```python
from build123d import *

# Parameters (mm, degrees)
ESQUISSE1_R             = 2
BOSS_EXTRU_1_DEPTH      = 5
ESQUISSE2_W             = 12
ESQUISSE2_H             = 2.5
BOSS_EXTRU_2_DEPTH      = 10
BOSS_EXTRU_2_2_DEPTH    = 10
ESQUISSE5_W             = 1.920676926
ESQUISSE5_H             = 10
BOSS_EXTRU_4_DEPTH      = 6.1
ESQUISSE7_W             = 2.5
ESQUISSE7_H             = 10
BOSS_EXTRU_6_DEPTH      = 1.920676926
CONG_4_RADIUS           = 5
CONG_4_LENGTH           = 2.5
BOSS_EXTRU_5_DEPTH      = 10
ESQUISSE4_R             = 2
ENL_V_MAT_EXTRU_2_DEPTH = 27.8404319
CONG_5_RADIUS           = 5
CONG_5_LENGTH           = 2.5


with BuildPart() as part:
    # Esquisse1 → Boss.-Extru.1 (new body)
    with BuildSketch(Plane.XY):
        with BuildLine():
            Line((-15, 5), (10, 5))
            Line((10, 5), (10, -5))
            Line((10, -5), (-15, -5))
            ThreePointArc((-15, -5), (-20, 0), (-15, 5))
        make_face()
        with Locations((-15, 0)):
            Circle(ESQUISSE1_R, mode=Mode.SUBTRACT)
    extrude(amount=BOSS_EXTRU_1_DEPTH)

    # Esquisse5 → Boss.-Extru.4 (add)
    with BuildSketch(Plane.XY.offset(-0.55)):
        with Locations((10.960338463, 0)):
            Rectangle(ESQUISSE5_W, ESQUISSE5_H)
    extrude(amount=BOSS_EXTRU_4_DEPTH)



with BuildPart() as body_2:
    # Esquisse2 → Boss.-Extru.2 (new, through all)
    with BuildSketch(Plane(origin=(0, 5, 0), x_dir=(1, 0, 0), z_dir=(0, 1, 0))):
        with Locations((17.920676926, 1.8)):
            Rectangle(ESQUISSE2_W, ESQUISSE2_H)
    extrude(amount=-BOSS_EXTRU_2_DEPTH)


with BuildPart() as body_3:
    # Esquisse2 → Boss.-Extru.2 2 (new, through all)
    with BuildSketch(Plane(origin=(0, 5, 0), x_dir=(1, 0, 0), z_dir=(0, 1, 0))):
        with Locations((17.920676926, -6.8)):
            Rectangle(ESQUISSE2_W, ESQUISSE2_H)
    extrude(amount=-BOSS_EXTRU_2_2_DEPTH)


with BuildPart() as part_1:
    add(part.part)

    add(body_2.part)  # Boss.-Extru.6 merges body 2

    add(body_3.part)  # Boss.-Extru.6 merges body 3
    # Esquisse7 → Boss.-Extru.6 (add)
    with BuildSketch(Plane.ZY.offset(-11.920676926)):
        with Locations((-1.8, 0)):
            Rectangle(ESQUISSE7_W, ESQUISSE7_H)
        with Locations((6.8, 0)):
            Rectangle(ESQUISSE7_W, ESQUISSE7_H)
    extrude(amount=BOSS_EXTRU_6_DEPTH)

    # Congé4: full round fillet: the end face becomes a half cylinder, R = half its width
    cong_4_face = Plane((23.920676926, 0, 6.8), x_dir=(0, 0, 1), z_dir=(1, 0, 0))  # on the end face: x along it, z out of the body
    cong_4_slab = cong_4_face.offset(-CONG_4_RADIUS / 2) * Box(CONG_4_LENGTH, 2 * CONG_4_RADIUS, CONG_4_RADIUS, mode=Mode.PRIVATE)  # the body's end, R deep
    cong_4_round = Plane((18.920676926, 0, 6.8), x_dir=(1, 0, 0), z_dir=(0, 0, 1)) * Cylinder(CONG_4_RADIUS, CONG_4_LENGTH, mode=Mode.PRIVATE)  # its axis R under the face
    add(cong_4_slab - cong_4_round, mode=Mode.SUBTRACT)

    # Esquisse6 → Boss.-Extru.5 (add, through all)
    with BuildSketch(Plane(origin=(0, 5, 0), x_dir=(1, 0, 0), z_dir=(0, 1, 0))):
        Polygon((10, 0), (10, 3.05), (4.799024164, 0), align=None)
        Polygon((4.799024164, -5), (10, -8.05), (10, -5), align=None)
    extrude(amount=-BOSS_EXTRU_5_DEPTH)

    # Esquisse4 → Enlèv. mat.-Extru.2 (cut, through all)
    with BuildSketch(Plane(origin=(0, 0, -3.05), x_dir=(-1, 0, 0), z_dir=(0, 0, -1))):
        with Locations((-18.856076392, 0)):
            Circle(ESQUISSE4_R)
    extrude(amount=-ENL_V_MAT_EXTRU_2_DEPTH, mode=Mode.SUBTRACT)

    # Congé5: full round fillet: the end face becomes a half cylinder, R = half its width
    cong_5_face = Plane((23.920676926, 0, -1.8), x_dir=(0, 0, -1), z_dir=(1, 0, 0))  # on the end face: x along it, z out of the body
    cong_5_slab = cong_5_face.offset(-CONG_5_RADIUS / 2) * Box(CONG_5_LENGTH, 2 * CONG_5_RADIUS, CONG_5_RADIUS, mode=Mode.PRIVATE)  # the body's end, R deep
    cong_5_round = Plane((18.920676926, 0, -1.8), x_dir=(1, 0, 0), z_dir=(0, 0, -1)) * Cylinder(CONG_5_RADIUS, CONG_5_LENGTH, mode=Mode.PRIVATE)  # its axis R under the face
    add(cong_5_slab - cong_5_round, mode=Mode.SUBTRACT)


solid = part_1.part
```
Geometry: final body of the model. Coordinates: model frame, mm. A direction names the side the tool comes from. Round coordinates to 2 decimals unless told otherwise and drop trailing zeros. Write each loop counter-clockwise with the first axis right and the second up, starting at its lowest first coordinate (ties: lowest second). Pieces come first, ordered by that corner, then holes. Notation, with made-up numbers: (85.25, 46.5) -> (131.25, 46.5) arc R7 ccw to (131.25, 56.5) -> close; hole circle Ø7 at (8.5, 24.25). An arc over 180 degrees is marked (long way). Return JSON: item names as keys, results as strings.
Q1. Set-up query: faces 4 (the flat face through (16.5, 0.1, -0.55)), 5 (the flat face through (-7, 0, 5)), 6 (the flat face through (-7, 0, 0)). Return all of +Z, -Z, +X, -X, +Y, -Y with unobstructed straight access to the full face (end or side cutting, diameter ignored); none if empty.
From the geometry:
{"face 4": "+X, +Y, -Y", "face 5": "+Z, -X, +Y, -Y", "face 6": "-Z, -X, +Y, -Y"}
Q2. Section D-D on y = 4. Return the cut outline in (x, z), and give its area (3 significant figures).
From the geometry:
{"outline": "(-18, 0) -> (4.8, 0) -> (10, -3.05) -> (21.92, -3.05) -> (21.92, -0.55) -> (11.92, -0.55) -> (11.92, 5.55) -> (21.92, 5.55) -> (21.92, 8.05) -> (10, 8.05) -> (4.8, 5) -> (-18, 5) -> close", "area": "227 mm2"}
Q3. Ray query, line 1 (Z direction, x = 18, y = -2.25); line 2 (Y direction, x = -15, z = 2.95); line 3 (Z direction, x = 4, y = 1). Return the intervals inside material, ascending.
From the geometry:
{"line 1": "-3.05 to -0.55, 5.55 to 8.05", "line 2": "-5 to -2, 2 to 5", "line 3": "0 to 5"}
Q4. Mould query, pull axis Y, two halves, no side actions, for faces 1 (the cylindrical face through (23.92, -0.11, 6.82)), 2 (the flat face through (7.36, 0.07, 6.5)), 3 (the cylindrical face through (16.95, 0.6, 6.78)). Classes: +Y half, -Y half, draft (parallel to the pull), parting line (faces both ways), or undercut.
From the geometry:
{"face 1": "parting line", "face 2": "draft", "face 3": "undercut"}
Q5. Section A-A on y = 0. Return the cut outline in (x, z), and give its area (3 significant figures).
From the geometry:
{"outline": "(-20, 0) -> (-17, 0) -> (-17, 5) -> (-20, 5) -> close; (-13, 0) -> (4.8, 0) -> (10, -3.05) -> (16.86, -3.05) -> (16.86, -0.55) -> (11.92, -0.55) -> (11.92, 5.55) -> (16.86, 5.55) -> (16.86, 8.05) -> (10, 8.05) -> (4.8, 5) -> (-13, 5) -> close; (20.86, -3.05) -> (23.92, -3.05) -> (23.92, -0.55) -> (20.86, -0.55) -> close; (20.86, 5.55) -> (23.92, 5.55) -> (23.92, 8.05) -> (20.86, 8.05) -> close", "area": "207 mm2"}
Q6. First-contact query: pin 1 Ø5 at (x, y) = (-5, -3) entering from -Z; pin 2 Ø1.5 at (y, z) = (-2, -1.5) entering from +X; pin 3 Ø5 at (y, z) = (2.5, 2.5) entering from +X. Flat tips, straight axial feed; report the tip coordinate or a pass-through.
From the geometry:
{"pin 1": "z = 0", "pin 2": "x = 23.76", "pin 3": "x = 11.92"}
Q7. Section C-C on z = 2.5. Return the cut outline in (x, y).
From the geometry:
{"outline": "(-15, -5) -> (11.92, -5) -> (11.92, 5) -> (-15, 5) arc R5 ccw to start; hole circle Ø4 at (-15, 0)"}
Q8. Section B-B on x = 15.5. Return the cut outline in (y, z).
From the geometry:
{"outline": "(-5, -3.05) -> (5, -3.05) -> (5, -0.55) -> (-5, -0.55) -> close; (-5, 5.55) -> (5, 5.55) -> (5, 8.05) -> (-5, 8.05) -> close"}
